Design review of the part built by this model. Coordinates are the model's own, in mm. Coordinates: 2 decimals unless noted, no trailing zeros. Write each loop counter-clockwise with the first axis right and the second up, starting at its lowest first coordinate (ties: lowest second). Pieces come first, ordered by that corner, then holes. Notation, with made-up numbers: (25, 88) - (68, 88) arc R23 cw to (68, 112) - close; hole circle Ø6 at (9, 23). An arc over 180 degrees is marked (long way). Use a Markdown table: item, result.
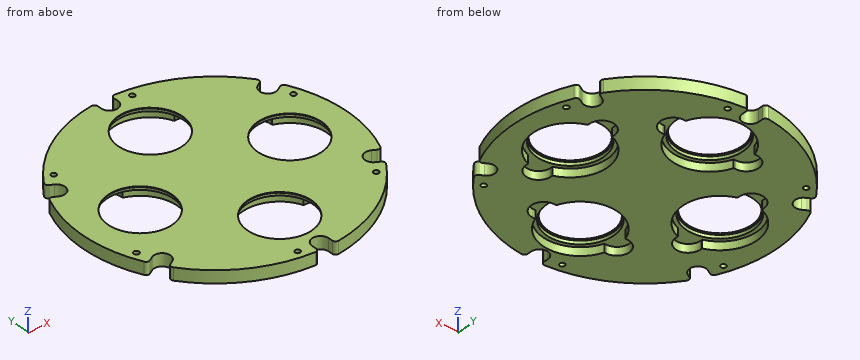
from build123d import *

# Parameters (mm, degrees)
BOSS_EXTRUDE1_DEPTH      = 9.525
F_10_32_TAPPED_HOLE1_D   = 4.0386
SUBSTRATE_CSINK_R        = 25.654
CUT_EXTRUDE1_DEPTH       = 9.017
SUBSTRATE_SURFACE_HOLE_R = 24.638
CUT_EXTRUDE2_DEPTH       = 144.717719729
CUT_EXTRUDE3_DEPTH       = 6.2992


with BuildPart() as part:
    # Front Plate Main → Boss-Extrude1 (new body)
    with BuildSketch(Plane.XY):
        with BuildLine():
            Line((-6.35, 98.660283296), (-6.35, 95.25))
            ThreePointArc((-6.35, 95.25), (0, 88.9), (6.35, 95.25))
            Line((6.35, 95.25), (6.35, 98.660283296))
            ThreePointArc((6.35, 98.660283296), (7.176434965, 100.53519526), (9.117948718, 101.190034149))
            ThreePointArc((9.117948718, 101.190034149), (50.8, 87.988181024), (83.074165824, 58.491392295))
            ThreePointArc((83.074165824, 58.491392295), (83.477815587, 56.482572618), (82.267311679, 54.829402962))
            Line((82.267311679, 54.829402962), (79.31391971, 53.124261314))
            ThreePointArc((79.31391971, 53.124261314), (76.989658396, 44.45), (85.66391971, 42.125738686))
            Line((85.66391971, 42.125738686), (88.617311679, 43.830880334))
            ThreePointArc((88.617311679, 43.830880334), (90.654250552, 44.052622641), (92.192114542, 42.698641855))
            ThreePointArc((92.192114542, 42.698641855), (101.6, 0), (92.192114542, -42.698641855))
            ThreePointArc((92.192114542, -42.698641855), (90.654250552, -44.052622641), (88.617311679, -43.830880334))
            Line((88.617311679, -43.830880334), (85.66391971, -42.125738686))
            ThreePointArc((85.66391971, -42.125738686), (76.989658396, -44.45), (79.31391971, -53.124261314))
            Line((79.31391971, -53.124261314), (82.267311679, -54.829402962))
            ThreePointArc((82.267311679, -54.829402962), (83.477815587, -56.482572618), (83.074165824, -58.491392295))
            ThreePointArc((83.074165824, -58.491392295), (50.8, -87.988181024), (9.117948718, -101.190034149))
            ThreePointArc((9.117948718, -101.190034149), (7.176434965, -100.53519526), (6.35, -98.660283296))
            Line((6.35, -98.660283296), (6.35, -95.25))
            ThreePointArc((6.35, -95.25), (0, -88.9), (-6.35, -95.25))
            Line((-6.35, -95.25), (-6.35, -98.660283296))
            ThreePointArc((-6.35, -98.660283296), (-7.176434965, -100.53519526), (-9.117948718, -101.190034149))
            ThreePointArc((-9.117948718, -101.190034149), (-50.8, -87.988181024), (-83.074165824, -58.491392295))
            ThreePointArc((-83.074165824, -58.491392295), (-83.477815587, -56.482572618), (-82.267311679, -54.829402962))
            Line((-82.267311679, -54.829402962), (-79.31391971, -53.124261314))
            ThreePointArc((-79.31391971, -53.124261314), (-76.989658396, -44.45), (-85.66391971, -42.125738686))
            Line((-85.66391971, -42.125738686), (-88.617311679, -43.830880334))
            ThreePointArc((-88.617311679, -43.830880334), (-90.654250552, -44.052622641), (-92.192114542, -42.698641855))
            ThreePointArc((-92.192114542, -42.698641855), (-101.6, 0), (-92.192114542, 42.698641855))
            ThreePointArc((-92.192114542, 42.698641855), (-90.654250552, 44.052622641), (-88.617311679, 43.830880334))
            Line((-88.617311679, 43.830880334), (-85.66391971, 42.125738686))
            ThreePointArc((-85.66391971, 42.125738686), (-76.989658396, 44.45), (-79.31391971, 53.124261314))
            Line((-79.31391971, 53.124261314), (-82.267311679, 54.829402962))
            ThreePointArc((-82.267311679, 54.829402962), (-83.477815587, 56.482572618), (-83.074165824, 58.491392295))
            ThreePointArc((-83.074165824, 58.491392295), (-50.8, 87.988181024), (-9.117948718, 101.190034149))
            ThreePointArc((-9.117948718, 101.190034149), (-7.176434965, 100.53519526), (-6.35, 98.660283296))
        make_face()
    extrude(amount=BOSS_EXTRUDE1_DEPTH)

    # #10-32 Tapped Hole1 (through all)
    with Locations(Plane(origin=(0, 0, 0), x_dir=(-1, 0, 0), z_dir=(0, 0, -1))):
        with Locations((-16.539988923, 93.802938474), (72.965733207, 61.225519823), (89.50572213, -32.577418652), (16.539988923, -93.802938474), (-72.965733207, -61.225519823), (-89.50572213, 32.577418652)):
            Hole(F_10_32_TAPPED_HOLE1_D / 2)

    # Substrate CSink → Cut-Extrude1 (cut)
    with BuildSketch(Plane(origin=(0, 0, 0), x_dir=(-1, 0, 0), z_dir=(0, 0, -1))):
        with Locations((0, 58.42)):
            Circle(SUBSTRATE_CSINK_R)
        with Locations((58.42, 0)):
            Circle(SUBSTRATE_CSINK_R)
        with Locations((0, -58.42)):
            Circle(SUBSTRATE_CSINK_R)
        with Locations((-58.42, 0)):
            Circle(SUBSTRATE_CSINK_R)
    extrude(amount=-CUT_EXTRUDE1_DEPTH, mode=Mode.SUBTRACT)

    # Substrate Surface Hole → Cut-Extrude2 (cut, through all)
    with BuildSketch(Plane(origin=(0, 0, 0), x_dir=(-1, 0, 0), z_dir=(0, 0, -1))):
        with Locations((0, 58.42)):
            Circle(SUBSTRATE_SURFACE_HOLE_R)
        with Locations((58.42, 0)):
            Circle(SUBSTRATE_SURFACE_HOLE_R)
        with Locations((0, -58.42)):
            Circle(SUBSTRATE_SURFACE_HOLE_R)
        with Locations((-58.42, 0)):
            Circle(SUBSTRATE_SURFACE_HOLE_R)
    extrude(amount=-CUT_EXTRUDE2_DEPTH, mode=Mode.SUBTRACT)

    # Backer Clearance → Cut-Extrude3 (cut)
    with BuildSketch(Plane(origin=(0, 0, 0), x_dir=(-1, 0, 0), z_dir=(0, 0, -1))):
        with BuildLine():
            Line((-28.575, 67.945), (-26.940768363, 67.945))
            ThreePointArc((-26.940768363, 67.945), (0, 86.995), (26.940768363, 67.945))
            Line((26.940768363, 67.945), (28.575, 67.945))
            ThreePointArc((28.575, 67.945), (38.1, 58.42), (28.575, 48.895))
            Line((28.575, 48.895), (26.940768363, 48.895))
            ThreePointArc((26.940768363, 48.895), (0, 29.845), (-26.940768363, 48.895))
            Line((-26.940768363, 48.895), (-28.575, 48.895))
            ThreePointArc((-28.575, 48.895), (-38.1, 58.42), (-28.575, 67.945))
        make_face()
        with BuildLine():
            Line((67.945, 28.575), (67.945, 26.940768363))
            ThreePointArc((67.945, 26.940768363), (86.995, 0), (67.945, -26.940768363))
            Line((67.945, -26.940768363), (67.945, -28.575))
            ThreePointArc((67.945, -28.575), (58.42, -38.1), (48.895, -28.575))
            Line((48.895, -28.575), (48.895, -26.940768363))
            ThreePointArc((48.895, -26.940768363), (29.845, 0), (48.895, 26.940768363))
            Line((48.895, 26.940768363), (48.895, 28.575))
            ThreePointArc((48.895, 28.575), (58.42, 38.1), (67.945, 28.575))
        make_face()
        with BuildLine():
            Line((28.575, -67.945), (26.940768363, -67.945))
            ThreePointArc((26.940768363, -67.945), (0, -86.995), (-26.940768363, -67.945))
            Line((-26.940768363, -67.945), (-28.575, -67.945))
            ThreePointArc((-28.575, -67.945), (-38.1, -58.42), (-28.575, -48.895))
            Line((-28.575, -48.895), (-26.940768363, -48.895))
            ThreePointArc((-26.940768363, -48.895), (0, -29.845), (26.940768363, -48.895))
            Line((26.940768363, -48.895), (28.575, -48.895))
            ThreePointArc((28.575, -48.895), (38.1, -58.42), (28.575, -67.945))
        make_face()
        with BuildLine():
            Line((-67.945, -28.575), (-67.945, -26.940768363))
            ThreePointArc((-67.945, -26.940768363), (-86.995, 0), (-67.945, 26.940768363))
            Line((-67.945, 26.940768363), (-67.945, 28.575))
            ThreePointArc((-67.945, 28.575), (-58.42, 38.1), (-48.895, 28.575))
            Line((-48.895, 28.575), (-48.895, 26.940768363))
            ThreePointArc((-48.895, 26.940768363), (-29.845, 0), (-48.895, -26.940768363))
            Line((-48.895, -26.940768363), (-48.895, -28.575))
            ThreePointArc((-48.895, -28.575), (-58.42, -38.1), (-67.945, -28.575))
        make_face()
    extrude(amount=-CUT_EXTRUDE3_DEPTH, mode=Mode.SUBTRACT)


solid = part.part
(1) Take a section at C-C on z = 2. State how many separate pieces and enclosed holes the cut face has, and give its area (3 significant figures).
Determined:
| item | result |
|---|---|
| separate pieces | 1 |
| enclosed holes | 10 |
| area | 20,000 mm2 |
(2) Take a section at B-B on x = -55. Write out the cut boundary in (y, z) (3 decimals), and give its area (3 significant figures).
Determined:
| item | result |
|---|---|
| outline | (-85.426, 0) - (-37.465, 0) - (-37.465, 6.299) - (-25.425, 6.299) - (-25.425, 9.017) - (-24.399, 9.017) - (-24.399, 9.525) - (-85.426, 9.525) - close; (24.399, 9.017) - (25.425, 9.017) - (25.425, 6.299) - (37.465, 6.299) - (37.465, 0) - (85.426, 0) - (85.426, 9.525) - (24.399, 9.525) - close |
| area | 992 mm2 |
(3) For pin 1 (3 mm diameter, centred on x = -51.5, z = 6.5, fed in from +Y); pin 2 (0.5 mm diameter, centred on x = -27.5, z = 2, fed in from +Y); pin 3 (0.5 mm diameter, centred on x = 28, z = 4.5, fed in from +Y), all flat-tipped, find the tip position at first contact; note any pin that passes through.
Determined:
| item | result |
|---|---|
| pin 1 | y = 88.45 |
| pin 2 | y = 97.88 |
| pin 3 | y = 97.74 |
(4) For L1, parallel to Y at x = 0, z = 7.55; L2, parallel to Y at x = 5, z = 0.75; L3, parallel to Y at x = -58.42, z = 9.4, list the stretches that pass through material, from the lowest coordinate up. Write a range as from..to.
Determined:
| item | result |
|---|---|
| L1 | -88.9..-84.07, -32.77..32.77, 84.07..88.9 |
| L2 | -91.34..-86.55, -30.29..30.29, 86.55..91.34 |
| L3 | -83.12..-24.64, 24.64..83.12 |
(5) Take a section at A-A on y = -74. Write out the cut boundary in (x, z) (1 decimal).
Determined:
| item | result |
|---|---|
| outline | (-69.6, 0) - (-24, 0) - (-24, 6.3) - (-20.4, 6.3) - (-20.4, 9) - (-19.1, 9) - (-19.1, 9.5) - (-69.6, 9.5) - close; (19.1, 9) - (20.4, 9) - (20.4, 6.3) - (24, 6.3) - (24, 0) - (69.6, 0) - (69.6, 9.5) - (19.1, 9.5) - close |
